Autodesk Inventor part; units mm, degrees
ref_plane "YZ Plane" through (0, 0, 0) normal (1, 0, 0) x (0, 1, 0)
ref_plane "XZ Plane" through (0, 0, 0) normal (0, 1, 0) x (-1, 0, 0)
ref_plane "XY Plane" through (0, 0, 0) normal (0, 0, 1) x (1, 0, 0)
sketch "Sketch1" plane through (0, 0, 0) normal (0, 1, 0) x (-1, 0, 0)
  circle A0 centre (0, 0) radius 50
  circle A1 centre (0, 0) radius 55
  dimension "d0" = 100
  dimension "d1" = 110
extrude "Extrusion1" add sketch "Sketch1" along normal mid plane 10
chamfer "Chamfer1" distance 2 angle 45 1 edges at (50, 5, 0)
chamfer "Chamfer2" distance 2 angle 45 1 edges at (50, -5, 0)
sketch "Sketch2" plane through (0, 0, 0) normal (0, 1, 0) x (-1, 0, 0)
  point P0 (0, 0)
properties part number "Ring"
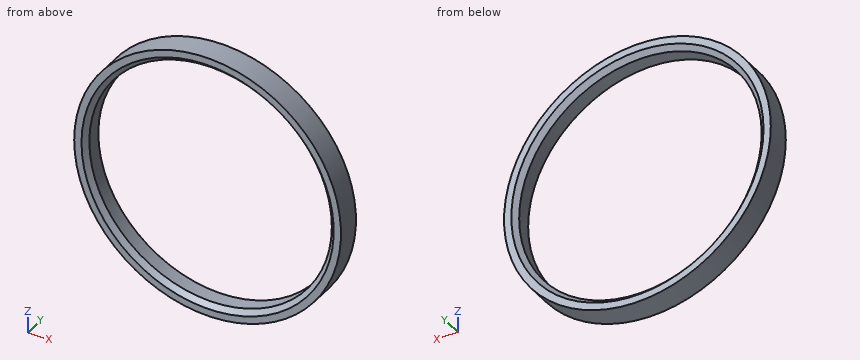
Verification items for the finished model (mm, model axes). Coordinates: 2 decimals unless noted, no trailing zeros. Loops run counter-clockwise (first coordinate to the right, second up) from the corner with the lowest first, then second, coordinate; pieces in that order, holes last. Notation, with made-up numbers: (79.25, -14) -> (128.25, -14) arc R27 ccw to (128.25, 13) -> close; hole circle Ø1 at (68, 11.25). An arc over 180 degrees is marked (long way). Answer as a JSON object with one key per item and string values. Group by question number.
Item 1: Scan lines: probe 1 along Z at (x, y) = (0, 1); probe 2 along X at (y, z) = (-3.25, 42); probe 3 along X at (y, z) = (3.5, 3.5). Record each from-to range of solid material in increasing order.
Item 2: Sectioned sample at A-A on x = 0. Record the boundary of the cut face in (y, z).
Item 3: Depth check by flat-ended pin: pin 1 (6 mm diameter, centred on y = -3, z = 9, fed in from +X); pin 2 (1 mm diameter, centred on x = 7.5, y = 3, fed in from -Z); pin 3 (2 mm diameter, centred on x = 22, y = 0.5, fed in from -Z). Enter the tip coordinate at first touch or a pass-through.
Item 4: Sectioned sample at C-C on y = -1. Record the boundary of the cut face in (x, z).
Item 5: Sectioned sample at B-B on z = 0. Record the boundary of the cut face in (x, y).
Evaluation:
{
 "1": {"probe 1": "z = -55 to -50, 50 to 55", "probe 2": "x = -35.51 to -27.59, 27.59 to 35.51", "probe 3": "x = -54.89 to -50.38, 50.38 to 54.89"},
 "2": {"outline": "(-5, -55) -> (5, -55) -> (5, -52) -> (3, -50) -> (-3, -50) -> (-5, -52) -> close; (-5, 52) -> (-3, 50) -> (3, 50) -> (5, 52) -> (5, 55) -> (-5, 55) -> close"},
 "3": {"pin 1": "stops at x = 54.67", "pin 2": "stops at z = -54.55", "pin 3": "stops at z = -50.83"},
 "4": {"outline": "circle Ø110 at (0, 0); hole circle Ø100 at (0, 0)"},
 "5": {"outline": "(-55, -5) -> (-52, -5) -> (-50, -3) -> (-50, 3) -> (-52, 5) -> (-55, 5) -> close; (50, -3) -> (52, -5) -> (55, -5) -> (55, 5) -> (52, 5) -> (50, 3) -> close"}
}
